Verification items for the finished model (mm, model axes). A direction names the side the tool comes from. Give positions to 0.01 mm unless a question says otherwise; leave off trailing zeros. Order: outer loops, then holes, each group sorted by start corner. A loop starts at its lowest first (then second) coordinate and runs counter-clockwise, first axis right, second up. Notation, with made-up numbers: (-27.75, -11) -> (29.25, -11) arc R22 cw to (29.25, 22) -> close; hole circle Ø4 at (83.25, 31). An arc over 180 degrees is marked (long way). Return JSON: item names as keys, results as strings. Group by question number.
(1) Release check for a two-part mould opening along Y. For faces 1 (the face through (10, 19, 24)), 2 (the face through (2, 8, 22)), 3 (the face through (10, 15, 26)) record: pulls with the +Y half, pulls with the -Y half, needs draft (parallel to the pull), parting line crosses it, or undercut.
(2) Depth check by flat-ended pin: pin 1 Ø0.5 at (x, z) = (9.5, 26) entering from +Y; pin 2 Ø3 at (x, z) = (2.5, 22) entering from +Y; pin 3 Ø5 at (x, z) = (15, -19.5) entering from +Y. Enter the tip coordinate at first touch or a pass-through.
(3) Cross-section at D-D on z = 22.5. Enter the section's corners in (x, y), then the cut area to 4 significant figures.
(4) Thickness scan on line 1 along X through (y, z) = (19, 26); line 2 along Z through (x, y) = (-17.5, 16.25); line 3 along X through (y, z) = (20.25, -26). Record the ranges inside material, lowest first.
(5) Cross-section at B-B on z = 12. Enter the section's corners in (x, y), then the cut area to 3 significant figures.
(6) Cross-section at C-C on x = 18.5. Enter the section's corners in (y, z), then the cut area to 3 significant figures.
(7) Tool access check on faces 4 (the face through (-7.5, 19, -26)), 5 (the face through (0, 0, 0)). Record the directions out of +Z, -Z, +X, -X, +Y, -Y that give a thin tool (end or side, any length) a straight path to the whole face; none if there is none.
(8) Cross-section at A-A on y = 13. Enter the section's corners in (x, z), then the cut area to 3 significant figures.
from build123d import *

# Parameters (mm, degrees)
SALIENTE_EXTRUIR1_DEPTH = 23
CROQUIS2_W              = 40
CROQUIS2_H              = 56
CORTAR_EXTRUIR1_DEPTH   = 20
CROQUIS3_R              = 2
SALIENTE_EXTRUIR2_DEPTH = 2
CROQUIS4_R              = 1.25
SALIENTE_EXTRUIR3_DEPTH = 3
CROQUIS5_W              = 4
CROQUIS5_H              = 8
SALIENTE_EXTRUIR4_DEPTH = 4
CROQUIS6_W              = 4
CROQUIS6_H              = 8
SALIENTE_EXTRUIR5_DEPTH = 4
CROQUIS7_R              = 0.5
CORTAR_EXTRUIR2_DEPTH   = 7
CORTAR_EXTRUIR3_REACH   = 58.993
CROQUIS9_W              = 5
CROQUIS9_H              = 9


with BuildPart() as part:
    # Croquis1 → Saliente-Extruir1 (new body)
    with BuildSketch(Plane(origin=(0, 0, 0), x_dir=(1, 0, 0), z_dir=(0, 1, 0))):
        with BuildLine():
            Line((-19.5, 29.5), (19.5, 29.5))
            ThreePointArc((19.5, 29.5), (20.914213562, 28.914213562), (21.5, 27.5))
            Line((21.5, 27.5), (21.5, -27.5))
            ThreePointArc((21.5, -27.5), (20.914213562, -28.914213562), (19.5, -29.5))
            Line((19.5, -29.5), (-19.5, -29.5))
            ThreePointArc((-19.5, -29.5), (-20.914213562, -28.914213562), (-21.5, -27.5))
            Line((-21.5, -27.5), (-21.5, 27.5))
            ThreePointArc((-21.5, 27.5), (-20.914213562, 28.914213562), (-19.5, 29.5))
        make_face()
    extrude(amount=SALIENTE_EXTRUIR1_DEPTH)

    # Croquis2 → Cortar-Extruir1 (cut)
    with BuildSketch(Plane(origin=(0, 23, 0), x_dir=(1, 0, 0), z_dir=(0, 1, 0))):
        Rectangle(CROQUIS2_W, CROQUIS2_H)
    extrude(amount=-CORTAR_EXTRUIR1_DEPTH, mode=Mode.SUBTRACT)

    # Croquis3 → Saliente-Extruir2 (add)
    with BuildSketch(Plane(origin=(0, 3, 0), x_dir=(1, 0, 0), z_dir=(0, 1, 0))):
        with Locations(Location((-16, 20.5, 0), (0, 0, 270))):
            Circle(CROQUIS3_R)
        with Locations(Location((2, -22.5, 0), (0, 0, 270))):
            Circle(CROQUIS3_R)
    extrude(amount=SALIENTE_EXTRUIR2_DEPTH)

    # Croquis4 → Saliente-Extruir3 (add)
    with BuildSketch(Plane(origin=(0, 5, 0), x_dir=(1, 0, 0), z_dir=(0, 1, 0))):
        with Locations(Location((-16, 20.5, 0), (0, 0, 270))):
            Circle(CROQUIS4_R)
        with Locations(Location((2, -22.5, 0), (0, 0, 270))):
            Circle(CROQUIS4_R)
    extrude(amount=SALIENTE_EXTRUIR3_DEPTH)

    # Croquis5 → Saliente-Extruir4 (add)
    with BuildSketch(Plane.XY.offset(-28)):
        with Locations((-9.5, 19)):
            Rectangle(CROQUIS5_W, CROQUIS5_H)
    extrude(amount=SALIENTE_EXTRUIR4_DEPTH)

    # Croquis6 → Saliente-Extruir5 (add)
    with BuildSketch(Plane(origin=(0, 0, 28), x_dir=(-1, 0, 0), z_dir=(0, 0, -1))):
        with Locations((-9.5, 19)):
            Rectangle(CROQUIS6_W, CROQUIS6_H)
    extrude(amount=SALIENTE_EXTRUIR5_DEPTH)

    # Croquis7 → Cortar-Extruir2 (cut)
    with BuildSketch(Plane(origin=(0, 23, 0), x_dir=(1, 0, 0), z_dir=(0, 1, 0))):
        with Locations(Location((-9.5, 26, 0), (0, 0, 270))):
            Circle(CROQUIS7_R)
        with Locations(Location((9.5, -26, 0), (0, 0, 270))):
            Circle(CROQUIS7_R)
    extrude(amount=-CORTAR_EXTRUIR2_DEPTH, mode=Mode.SUBTRACT)

    # Croquis9 → Cortar-Extruir3 (cut, up to next)
    with BuildSketch(Plane.ZY.offset(21.5), mode=Mode.PRIVATE) as cortar_extruir3_sk1:
        with Locations((-23.5, 15.5)):
            Rectangle(CROQUIS9_W, CROQUIS9_H)
    cortar_extruir3_tool1 = extrude(cortar_extruir3_sk1.sketch, amount=-CORTAR_EXTRUIR3_REACH, mode=Mode.PRIVATE) & part.part
    add(cortar_extruir3_tool1.solids().sort_by_distance((-21.5, 15.5, -23.5))[0], mode=Mode.SUBTRACT)


solid = part.part
Verdict:
{
 "1": {"face 1": "needs draft", "face 2": "pulls with the +Y half", "face 3": "undercut"},
 "2": {"pin 1": "y = 16", "pin 2": "y = 8", "pin 3": "y = 3"},
 "3": {"outline": "(-21.5, 0) -> (21.5, 0) -> (21.5, 23) -> (20, 23) -> (20, 3) -> (4, 3) -> (4, 5) -> (3.25, 5) -> (3.25, 8) -> (0.75, 8) -> (0.75, 5) -> (0, 5) -> (0, 3) -> (-20, 3) -> (-20, 23) -> (-21.5, 23) -> close", "area": "204.5 mm²"},
 "4": {"line 1": "-21.5 to -20, 7.5 to 9, 10 to 11.5, 20 to 21.5", "line 2": "-29.5 to -28, 28 to 29.5", "line 3": "-21.5 to -20, -11.5 to -10, -9 to -7.5, 20 to 21.5"},
 "5": {"outline": "(-21.5, 0) -> (21.5, 0) -> (21.5, 23) -> (20, 23) -> (20, 3) -> (-20, 3) -> (-20, 23) -> (-21.5, 23) -> close", "area": "189 mm²"},
 "6": {"outline": "(0, -29.5) -> (23, -29.5) -> (23, -28) -> (3, -28) -> (3, 28) -> (23, 28) -> (23, 29.5) -> (0, 29.5) -> close", "area": "237 mm²"},
 "7": {"face 4": "+Y", "face 5": "+Z, -Z, +X, -X, -Y"},
 "8": {"outline": "(-21.5, -27.5) arc R2 ccw to (-19.5, -29.5) -> (19.5, -29.5) arc R2 ccw to (21.5, -27.5) -> (21.5, 27.5) arc R2 ccw to (19.5, 29.5) -> (-19.5, 29.5) arc R2 ccw to (-21.5, 27.5) -> (-21.5, -21) -> (-20, -21) -> (-20, 28) -> (20, 28) -> (20, -28) -> (-20, -28) -> (-20, -26) -> (-21.5, -26) -> close", "area": "286 mm²"}
}
